Here's the drawing with two shaded views (mm, measured from the low corner). I have some questions. Round coordinates to 2 decimals unless told otherwise and drop trailing zeros. Loops run counter-clockwise (first coordinate to the right, second up) from the corner with the lowest first, then second, coordinate; pieces in that order, holes last. Notation, with made-up numbers: (48, 14) -> (104, 14) arc R17 ccw to (104, 31) -> close; hole circle Ø7 at (70, -6). An arc over 180 degrees is marked (long way). Use a Markdown table: item, result.
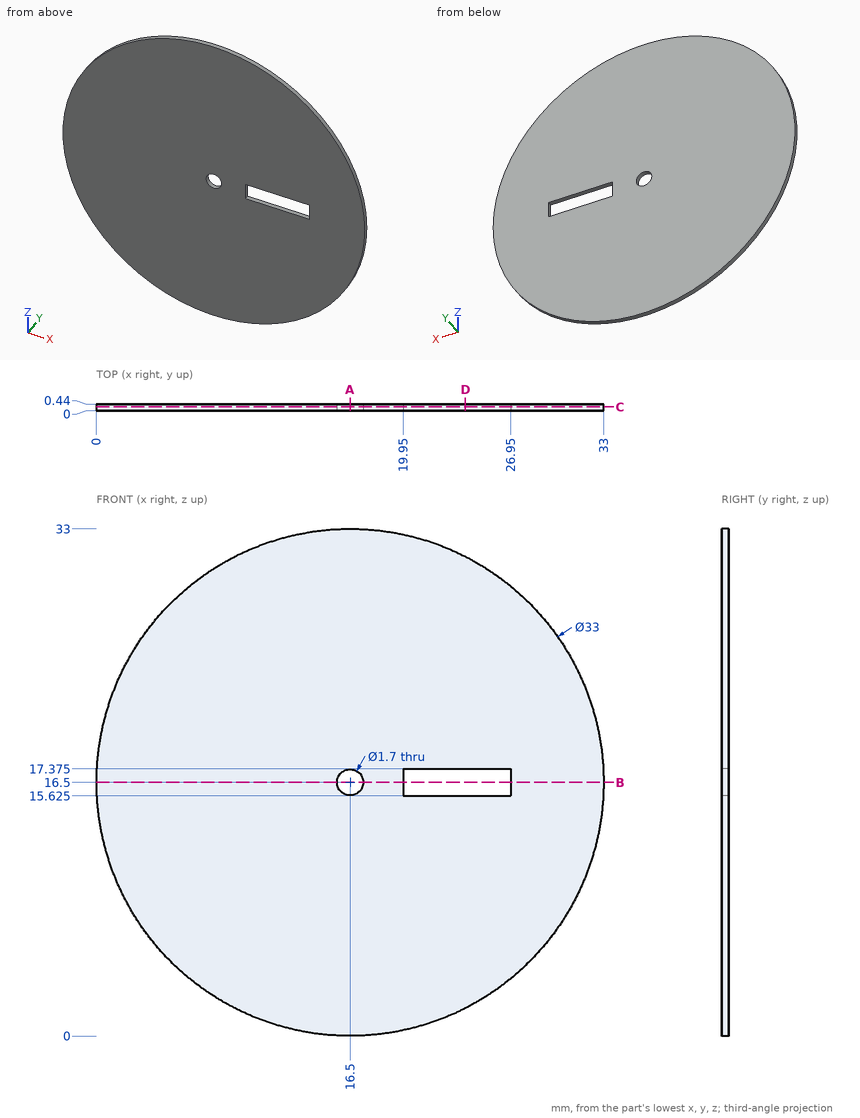
1. I want a section at C-C (y = 0.25). Please give me the cut outline in (x, z) (3 decimals).
Answer sheet:
| item | result |
|---|---|
| outline | circle Ø33 at (16.5, 16.5); hole circle Ø1.7 at (16.5, 16.5); hole (19.95, 15.625) -> (26.95, 15.625) -> (26.95, 17.375) -> (19.95, 17.375) -> close |
2. Will this pin go through, and if not, where does the flat tip stop? pin 1 Ø1 at (x, z) = (16.5, 16.5) entering from -Y.
Answer sheet:
| item | result |
|---|---|
| pin 1 | passes through |
3. I want a section at A-A (x = 16.5). Please give me the cut outline in (y, z), plus the area to 3 significant figures.
Answer sheet:
| item | result |
|---|---|
| outline | (0, 0) -> (0.44, 0) -> (0.44, 15.65) -> (0, 15.65) -> close; (0, 17.35) -> (0.44, 17.35) -> (0.44, 33) -> (0, 33) -> close |
| area | 13.8 mm² |
4. I want a section at B-B (z = 16.5). Please give me the cut outline in (x, y), plus the area to 3 significant figures.
Answer sheet:
| item | result |
|---|---|
| outline | (0, 0) -> (15.65, 0) -> (15.65, 0.44) -> (0, 0.44) -> close; (17.35, 0) -> (19.95, 0) -> (19.95, 0.44) -> (17.35, 0.44) -> close; (26.95, 0) -> (33, 0) -> (33, 0.44) -> (26.95, 0.44) -> close |
| area | 10.7 mm² |
5. I need wall thicknesses on line 1 (X direction, y = 0.3, z = 16.5); line 2 (Z direction, x = 16.5, y = 0.2); line 3 (X direction, y = 0.3, z = 17). Which ranges of each line are inside material? Lowest first, please.
Answer sheet:
| item | result |
|---|---|
| line 1 | x = 0 to 15.65, 17.35 to 19.95, 26.95 to 33 |
| line 2 | z = 0 to 15.65, 17.35 to 33 |
| line 3 | x = 0.01 to 15.81, 17.19 to 19.95, 26.95 to 32.99 |
6. I want a section at D-D (x = 24). Please give me the cut outline in (y, z) (3 decimals), plus the area to 3 significant figures.
Answer sheet:
| item | result |
|---|---|
| outline | (0, 1.803) -> (0.44, 1.803) -> (0.44, 15.625) -> (0, 15.625) -> close; (0, 17.375) -> (0.44, 17.375) -> (0.44, 31.197) -> (0, 31.197) -> close |
| area | 12.2 mm² |
